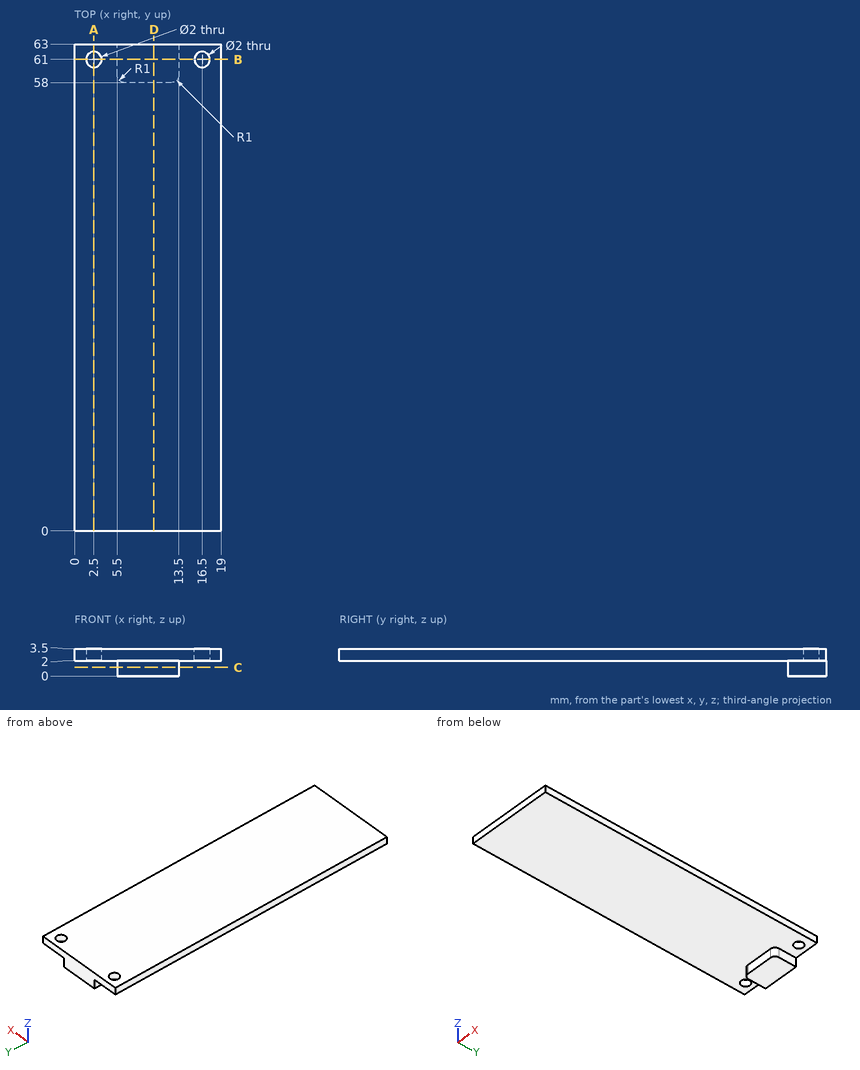
Geometry check sheet. Reference: drawing and pictorial views, mm from the part's lowest x, y, z. Coordinates: 2 decimals unless noted, no trailing zeros. Order: outer loops, then holes, each group sorted by start corner. A loop starts at its lowest first (then second) coordinate and runs counter-clockwise, first axis right, second up. Notation, with made-up numbers: (65.5, 87) - (92.5, 87) arc R15 ccw to (92.5, 116) - close; hole circle Ø9 at (88.5, 54.25). An arc over 180 degrees is marked (long way). One line per item, written item: value.
(1) Sectioned sample at A-A (x = 2.5). Enter the section's corners in (y, z).
Data:
outline: (0, 2) - (60, 2) - (60, 3.5) - (0, 3.5) - close; (62, 2) - (63, 2) - (63, 3.5) - (62, 3.5) - close
(2) Depth check by flat-ended pin: pin 1 Ø1.6 at (y, z) = (62, 0.5) entering from +X; pin 2 Ø1 at (x, y) = (8.5, 55) entering from -Z; pin 3 Ø1.8 at (x, y) = (16.5, 61) entering from +Z; pin 4 Ø2 at (x, z) = (8.5, 0.5) entering from -Y. Enter the tip coordinate at first touch or a pass-through.
Data:
pin 1: stops at x = 13.5
pin 2: stops at z = 2
pin 3: passes through
pin 4: stops at y = 58
(3) Thickness scan on probe 1 along X at (y, z) = (61, 3); probe 2 along Z at (x, y) = (13.5, 43); probe 3 along Y at (x, z) = (16.5, 2.85). Record the ranges inside material, lowest first. Write a range as from..to.
Data:
probe 1: x = 0..1.5, 3.5..15.5, 17.5..19
probe 2: z = 2..3.5
probe 3: y = 0..60, 62..63
(4) Sectioned sample at C-C (z = 1.1). Enter the section's corners in (x, y), and give its area (3 significant figures).
Data:
outline: (5.5, 59) arc R1 ccw to (6.5, 58) - (12.5, 58) arc R1 ccw to (13.5, 59) - (13.5, 63) - (5.5, 63) - close
area: 39.6 mm^2
(5) Sectioned sample at D-D (x = 10.25). Enter the section's corners in (y, z), and give its area (4 significant figures).
Data:
outline: (0, 2) - (58, 2) - (58, 0) - (63, 0) - (63, 3.5) - (0, 3.5) - close
area: 104.5 mm^2
(6) Sectioned sample at B-B (y = 61). Enter the section's corners in (x, z), and give its area (3 significant figures).
Data:
outline: (0, 2) - (1.5, 2) - (1.5, 3.5) - (0, 3.5) - close; (3.5, 2) - (5.5, 2) - (5.5, 0) - (13.5, 0) - (13.5, 2) - (15.5, 2) - (15.5, 3.5) - (3.5, 3.5) - close; (17.5, 2) - (19, 2) - (19, 3.5) - (17.5, 3.5) - close
area: 38.5 mm^2
